```python
from build123d import *

# Parameters (mm, degrees)
EXTRUDE_1_DEPTH     = 50
EXTRUDE_3_DEPTH     = 33.199998
EXTRUDE_4_REACH     = 79.048
SKETCH_4_W          = 50
SKETCH_4_H          = 2.121320344
CUT_EXTRUDE_1_DEPTH = 99.405896905
SKETCH_8_W          = 62
SKETCH_8_H          = 44.689148571
SKETCH_8_R          = 1.5
EXTRUDE_5_DEPTH     = 3
FILLET_1_R          = 10
FILLET_2_R          = 2
SKETCH_9_W          = 6.2
SKETCH_9_H          = 40
EXTRUDE_6_DEPTH     = 5
SKETCH_10_W         = 6.2
SKETCH_10_H         = 40
EXTRUDE_7_DEPTH     = 5


with BuildPart() as part:
    # 草图1 → 凸台-拉伸1 (new body)
    with BuildSketch(Plane.XY):
        Polygon((25.716046069, 61.209761814), (43.929249505, 61.209761814), (58.626662914, 46.512348406), (58.626662914, 1.823199835), (32.150717778, 1.823199835), (32.150717778, 4.823199835), (55.626662914, 28.29914497), (25.716046069, 58.209761814), align=None)
    extrude(amount=EXTRUDE_1_DEPTH)

    # 草图3 → 凸台-拉伸3 (add)
    with BuildSketch(Plane(origin=(41.962903942, 41.962903942, 0), x_dir=(0, 0, 1), z_dir=(-0.7071067811865476, -0.7071067811865476, 0))):
        Polygon((50, -19.323473251), (46.15, -19.323473251), (43.15, -19.323473251), (46.15, -16.323473251), (46.15, 19.976526749), (43.15, 22.976526749), (46.15, 22.976526749), (50, 22.976526749), align=None)
        Polygon((0, 22.976526749), (0, -19.323473251), (3.85, -19.323473251), (6.85, -19.323473251), (3.85, -16.323473251), (3.85, 19.976526749), (6.85, 22.976526749), (3.85, 22.976526749), align=None)
    extrude(amount=EXTRUDE_3_DEPTH)

    # 凸台-拉伸4: up to this plane
    extrude_4_end = Plane(origin=(25.716046069, 61.209761814, 50), z_dir=(0, -1, 0))
    # 草图4 → 凸台-拉伸4 (add, up to the surface)
    with BuildSketch(Plane(origin=(18.486958806, 18.486958806, 0), x_dir=(0, 0, 1), z_dir=(-0.7071067811865477, -0.7071067811865475, 0)), mode=Mode.PRIVATE) as extrude_4_sk1:
        with Locations((25, 24.037186921)):
            Rectangle(SKETCH_4_W, SKETCH_4_H)
    extrude_4_tool1 = split(extrude(extrude_4_sk1.sketch, amount=-EXTRUDE_4_REACH, mode=Mode.PRIVATE), bisect_by=extrude_4_end, keep=Keep.BOTH, mode=Mode.PRIVATE)
    add(extrude_4_tool1.solids().sort_by_distance((1.490101, 35.483817, 25))[0])

    # 草图5 → 切除-拉伸1 (cut, through all)
    with BuildSketch(Plane(origin=(0, 0, 0), x_dir=(-1, 0, 0), z_dir=(0, 0, -1))):
        Polygon((-35.014500242, 48.911307642), (-46.328208741, 37.597599143), (-22.852263606, 14.121654007), (-11.538555107, 25.435362506), align=None)
    extrude(amount=-CUT_EXTRUDE_1_DEPTH, mode=Mode.SUBTRACT)

    # 草图8 → 凸台-拉伸5 (add)
    with BuildSketch(Plane(origin=(58.626662914, 0, 0), x_dir=(0, 0, -1), z_dir=(1, 0, 0))):
        with Locations((-25, 24.16777412)):
            Rectangle(SKETCH_8_W, SKETCH_8_H)
        with Locations(Location((-53, 39.162348406, 0), (0, 0, 90))):
            Circle(SKETCH_8_R, mode=Mode.SUBTRACT)
        with Locations(Location((-53, 33.162348406, 0), (0, 0, 90))):
            Circle(SKETCH_8_R, mode=Mode.SUBTRACT)
        with Locations(Location((-53, 27.162348406, 0), (0, 0, 90))):
            Circle(SKETCH_8_R, mode=Mode.SUBTRACT)
        with Locations(Location((-53, 21.162348406, 0), (0, 0, 90))):
            Circle(SKETCH_8_R, mode=Mode.SUBTRACT)
        with Locations(Location((-53, 15.162348406, 0), (0, 0, 90))):
            Circle(SKETCH_8_R, mode=Mode.SUBTRACT)
        with Locations(Location((-53, 9.162348406, 0), (0, 0, 90))):
            Circle(SKETCH_8_R, mode=Mode.SUBTRACT)
        with Locations(Location((3, 9.162348406, 0), (0, 0, 270))):
            Circle(SKETCH_8_R, mode=Mode.SUBTRACT)
        with Locations(Location((3, 15.162348406, 0), (0, 0, 270))):
            Circle(SKETCH_8_R, mode=Mode.SUBTRACT)
        with Locations(Location((3, 21.162348406, 0), (0, 0, 270))):
            Circle(SKETCH_8_R, mode=Mode.SUBTRACT)
        with Locations(Location((3, 27.162348406, 0), (0, 0, 270))):
            Circle(SKETCH_8_R, mode=Mode.SUBTRACT)
        with Locations(Location((3, 33.162348406, 0), (0, 0, 270))):
            Circle(SKETCH_8_R, mode=Mode.SUBTRACT)
        with Locations(Location((3, 39.162348406, 0), (0, 0, 270))):
            Circle(SKETCH_8_R, mode=Mode.SUBTRACT)
    extrude(amount=-EXTRUDE_5_DEPTH)

    # 圆角1
    fillet_1_edges = [part.edges().sort_by_distance(p)[0] for p in [
        (25.716046069, 61.209761814, 25),
        (43.929249505, 61.209761814, 25),
    ]]
    fillet(fillet_1_edges, radius=FILLET_1_R)

    # 圆角2
    fillet_2_edges = [part.edges().sort_by_distance(p)[0] for p in [
        (52.742422303, 52.396589016, 0),
        (57.126662914, 1.823199835, -6),
        (57.126662914, 1.823199835, 56),
        (57.126662914, 46.512348406, 56),
        (57.126662914, 46.512348406, -6),
        (34.822647787, 61.209761814, 0),
        (34.822647787, 61.209761814, 50),
        (11.763607408, 47.257323152, 0),
        (26.031347369, 60.448557139, 0),
        (43.613948205, 60.448557139, 0),
        (11.763607408, 47.257323152, 50),
        (26.031347369, 60.448557139, 50),
        (43.613948205, 60.448557139, 50),
        (43.888690346, 1.823199835, 50),
        (43.888690346, 1.823199835, 0),
        (52.742422303, 52.396589016, 50),
    ]]
    fillet(fillet_2_edges, radius=FILLET_2_R)

    # 草图9 → 凸台-拉伸6 (add)
    with BuildSketch(Plane(origin=(58.626662914, 0, 0), x_dir=(0, 0, -1), z_dir=(1, 0, 0))):
        with Locations((-34.99740251, 23.658233783)):
            Rectangle(SKETCH_9_W, SKETCH_9_H)
    extrude(amount=EXTRUDE_6_DEPTH)

    # 草图10 → 凸台-拉伸7 (add)
    with BuildSketch(Plane(origin=(58.626662914, 0, 0), x_dir=(0, 0, -1), z_dir=(1, 0, 0))):
        with Locations((-14.997806006, 23.541157616)):
            Rectangle(SKETCH_10_W, SKETCH_10_H)
    extrude(amount=EXTRUDE_7_DEPTH)


solid = part.part
```
Work out the finished part from the listing and answer in its coordinate system (mm). A direction names the side the tool comes from. Give positions to 0.01 mm unless a question says otherwise; leave off trailing zeros. Loops run counter-clockwise (first coordinate to the right, second up) from the corner with the lowest first, then second, coordinate; pieces in that order, holes last. Notation, with made-up numbers: (3.5, -17) -> (44.5, -17) arc R16 cw to (44.5, -13) -> close; hole circle Ø11 at (-17.5, 19.25). An arc over 180 degrees is marked (long way). One line per question, with ' | ' between items. Start each with the question number.
1) Section C-C, the plane y = 9.5 is taken. State how many separate pieces and enclosed holes the cut face has, then the cut area to 3 significant figures.
2) Determine the mould class of faces 6 (the face through (35, 61.21, 25)), 7 (the face through (13.814, 46.307, 24.65)), 8 (the face through (57.106, 2.394, 55.399)) for opening direction Z: +Z half, -Z half, draft (parallel to the pull), parting line (faces both ways), or undercut.
3) Straight lines are drawn through the part: L1, parallel to Z at x = 21, y = 40; L2, parallel to Y at x = 55, z = 36; L3, parallel to X at y = 12, z = -3. For each, find the intervals that lie inside material, in ascending order.
4) Each of these flat-tipped pins is pushed along its axis until it touches: pin 1 (5 mm diameter, centred on y = 48.5, z = 9.5, fed in from -X); pin 2 (5 mm diameter, centred on y = 33, z = 5.5, fed in from +X); pin 3 (6 mm diameter, centred on x = 43, y = 15.5, fed in from +Z). Where does it stop, or does it pass through?
5) Section B-B, the plane z = 31 is taken. Determine the outline of the cut face in (x, y).
6) Section A-A, the plane z = 53 is taken. Determine the outline of the cut face in (x, y), then the cut area to 3 significant figures.
7) For faces 1 (the face through (61, 3.658, 35)), 2 (the face through (6.824, 30.15, 48.145)), 3 (the face through (43.007, 17.771, 5.371)), 4 (the face through (23.112, 37.009, 1.898)), 5 (the face through (43.724, 2.425, 49.43)), determine the directions among +Z, -Z, +X, -X, +Y, -Y from which every point of the face is accessible in a straight line to the end or side of a thin tool.
Resolved:
1) separate pieces: 3 | enclosed holes: 0 | area: 1,260 mm2
2) face 6: draft | face 7: undercut | face 8: +Z half
3) L1: 0 to 3.85, 46.15 to 50 | L2: 1.82 to 27.67, 28.93 to 50.14 | L3: 55.63 to 58.63
4) pin 1: x = 10.51 | pin 2: x = 58.63 | pin 3: z = 50
5) outline: (0.74, 36.23) -> (2.24, 34.73) -> (25.72, 58.21) -> (55.63, 28.3) -> (32.15, 4.82) -> (32.15, 1.82) -> (58.63, 1.82) -> (58.63, 46.51) -> (46.86, 58.28) arc R10 ccw to (39.79, 61.21) -> (29.86, 61.21) arc R10 ccw to (22.79, 58.28) -> close
6) outline: (55.63, 1.82) -> (58.63, 1.82) -> (58.63, 7.66) -> (55.63, 7.66) -> close; (55.63, 10.66) -> (58.63, 10.66) -> (58.63, 13.66) -> (55.63, 13.66) -> close; (55.63, 16.66) -> (58.63, 16.66) -> (58.63, 19.66) -> (55.63, 19.66) -> close; (55.63, 22.66) -> (58.63, 22.66) -> (58.63, 25.66) -> (55.63, 25.66) -> close; (55.63, 28.66) -> (58.63, 28.66) -> (58.63, 31.66) -> (55.63, 31.66) -> close; (55.63, 34.66) -> (58.63, 34.66) -> (58.63, 37.66) -> (55.63, 37.66) -> close; (55.63, 40.66) -> (58.63, 40.66) -> (58.63, 46.51) -> (55.63, 46.51) -> close | area: 80.1 mm2
7) face 1: +Z, +X, -Y | face 2: +Z, -Z, -X, -Y | face 3: -X | face 4: +Z, -Z | face 5: +Z, -X, -Y
